from build123d import *

# Parameters (mm, degrees)
CYLINDER1852_R              = 3
CYLINDER1852_DEPTH          = 3
CYLINDER1853_R              = 3
CYLINDER1853_DEPTH          = 3
CYLINDER1854_R              = 3
CYLINDER1854_DEPTH          = 3
CYLINDER1851_R              = 3
CYLINDER1851_DEPTH          = 3
COMPOUND933_ROLL_ANGLE      = 90
COMPOUND933_PLACEMENT_ANGLE = 45
CYLINDER1848_R              = 1.5
CYLINDER1848_DEPTH          = 40
CYLINDER1850_R              = 1.5
CYLINDER1850_DEPTH          = 40
CYLINDER1849_R              = 1.5
CYLINDER1849_DEPTH          = 40
CYLINDER1847_R              = 1.5
CYLINDER1847_DEPTH          = 40
COMPOUND925_ROLL_ANGLE      = 90
COMPOUND925_PLACEMENT_ANGLE = 45
CYLINDER1867_R              = 12
CYLINDER1867_DEPTH          = 20
CYLINDER1866_R              = 2.5
CYLINDER1866_DEPTH          = 20
CYLINDER1864_R              = 2.5
CYLINDER1864_DEPTH          = 20
CYLINDER1863_R              = 2.5
CYLINDER1863_DEPTH          = 20
CYLINDER1865_R              = 2.5
CYLINDER1865_DEPTH          = 20
BOX324_W                    = 20
BOX324_H                    = 8
BOX324_DEPTH                = 3
BOX328_W                    = 20
BOX328_H                    = 8
BOX328_DEPTH                = 3
BOX330_W                    = 20
BOX330_H                    = 8
BOX330_DEPTH                = 3
BOX323_W                    = 20
BOX323_H                    = 8
BOX323_DEPTH                = 3
BOX329_W                    = 68
BOX329_H                    = 65
BOX329_DEPTH                = 8
CHAMFER014_SIZE             = 4


with BuildPart() as obj1:
    # Cylinder1852 → Cylinder1852 (new body)
    with BuildSketch(Plane(origin=(16, 140, 49), x_dir=(1, 0, 0), z_dir=(0, -1, 0))):
        Circle(CYLINDER1852_R)
    extrude(amount=CYLINDER1852_DEPTH)


with BuildPart() as obj2:
    # Cylinder1853 → Cylinder1853 (new body)
    with BuildSketch(Plane(origin=(-16, 140, 49), x_dir=(1, 0, 0), z_dir=(0, -1, 0))):
        Circle(CYLINDER1853_R)
    extrude(amount=CYLINDER1853_DEPTH)


with BuildPart() as obj3:
    # Cylinder1854 → Cylinder1854 (new body)
    with BuildSketch(Plane(origin=(0, 140, 33), x_dir=(1, 0, 0), z_dir=(0, -1, 0))):
        Circle(CYLINDER1854_R)
    extrude(amount=CYLINDER1854_DEPTH)


with BuildPart() as compound933:
    # Cylinder1851 → Cylinder1851 (new body)
    with BuildSketch(Plane(origin=(0, 140, 65), x_dir=(1, 0, 0), z_dir=(0, -1, 0))):
        Circle(CYLINDER1851_R)
    extrude(amount=CYLINDER1851_DEPTH)

    # Compound933: union obj1, obj2, obj3
    add(obj1.part)
    add(obj2.part)
    add(obj3.part)


with BuildPart() as compound933_1:
    # Compound933 roll: moved
    add(compound933.part.rotate(Axis((0, 0, 0), (1, 0, 0)), COMPOUND933_ROLL_ANGLE))


with BuildPart() as compound933_2:
    # Compound933 placement: moved
    add(compound933_1.part.moved(Location((-34.65, 34.65, -167))).rotate(Axis((-34.65, 34.65, -167), (0, 0, 1)), COMPOUND933_PLACEMENT_ANGLE))


with BuildPart() as obj4:
    # Cylinder1848 → Cylinder1848 (new body)
    with BuildSketch(Plane(origin=(16, 140, 49), x_dir=(1, 0, 0), z_dir=(0, -1, 0))):
        Circle(CYLINDER1848_R)
    extrude(amount=CYLINDER1848_DEPTH)


with BuildPart() as obj5:
    # Cylinder1850 → Cylinder1850 (new body)
    with BuildSketch(Plane(origin=(-16, 140, 49), x_dir=(1, 0, 0), z_dir=(0, -1, 0))):
        Circle(CYLINDER1850_R)
    extrude(amount=CYLINDER1850_DEPTH)


with BuildPart() as obj6:
    # Cylinder1849 → Cylinder1849 (new body)
    with BuildSketch(Plane(origin=(0, 140, 33), x_dir=(1, 0, 0), z_dir=(0, -1, 0))):
        Circle(CYLINDER1849_R)
    extrude(amount=CYLINDER1849_DEPTH)


with BuildPart() as compound925:
    # Cylinder1847 → Cylinder1847 (new body)
    with BuildSketch(Plane(origin=(0, 140, 65), x_dir=(1, 0, 0), z_dir=(0, -1, 0))):
        Circle(CYLINDER1847_R)
    extrude(amount=CYLINDER1847_DEPTH)

    # Compound925: union obj4, obj5, obj6
    add(obj4.part)
    add(obj5.part)
    add(obj6.part)


with BuildPart() as compound925_1:
    # Compound925 roll: moved
    add(compound925.part.rotate(Axis((0, 0, 0), (1, 0, 0)), COMPOUND925_ROLL_ANGLE))


with BuildPart() as compound925_2:
    # Compound925 placement: moved
    add(compound925_1.part.moved(Location((-34.65, 34.65, -144))).rotate(Axis((-34.65, 34.65, -144), (0, 0, 1)), COMPOUND925_PLACEMENT_ANGLE))


with BuildPart() as obj7:
    # Cylinder1867 → Cylinder1867 (new body)
    with BuildSketch(Plane.XY.offset(-39)):
        Circle(CYLINDER1867_R)
    extrude(amount=CYLINDER1867_DEPTH)


with BuildPart() as obj8:
    # Cylinder1866 → Cylinder1866 (new body)
    with BuildSketch(Plane(origin=(-23.55, 23.55, -34), x_dir=(1, 0, 0), z_dir=(0, 0, 1))):
        Circle(CYLINDER1866_R)
    extrude(amount=CYLINDER1866_DEPTH)


with BuildPart() as obj9:
    # Cylinder1864 → Cylinder1864 (new body)
    with BuildSketch(Plane(origin=(-23.55, -23.55, -34), x_dir=(1, 0, 0), z_dir=(0, 0, 1))):
        Circle(CYLINDER1864_R)
    extrude(amount=CYLINDER1864_DEPTH)


with BuildPart() as obj10:
    # Cylinder1863 → Cylinder1863 (new body)
    with BuildSketch(Plane(origin=(23.55, -23.55, -34), x_dir=(1, 0, 0), z_dir=(0, 0, 1))):
        Circle(CYLINDER1863_R)
    extrude(amount=CYLINDER1863_DEPTH)


with BuildPart() as compound931:
    # Cylinder1865 → Cylinder1865 (new body)
    with BuildSketch(Plane(origin=(23.55, 23.55, -34), x_dir=(1, 0, 0), z_dir=(0, 0, 1))):
        Circle(CYLINDER1865_R)
    extrude(amount=CYLINDER1865_DEPTH)

    # Compound931: union obj8, obj9, obj10
    add(obj8.part)
    add(obj9.part)
    add(obj10.part)


with BuildPart() as krychle324:
    # Box324 → Box324 (new body)
    with BuildSketch(Plane(origin=(17.55, -27.55, -28), x_dir=(1, 0, 0), z_dir=(0, 0, 1))):
        with Locations((10, 4)):
            Rectangle(BOX324_W, BOX324_H)
    extrude(amount=BOX324_DEPTH)


with BuildPart() as krychle328:
    # Box328 → Box328 (new body)
    with BuildSketch(Plane(origin=(-37.45, 19.55, -28), x_dir=(1, 0, 0), z_dir=(0, 0, 1))):
        with Locations((10, 4)):
            Rectangle(BOX328_W, BOX328_H)
    extrude(amount=BOX328_DEPTH)


with BuildPart() as krychle330:
    # Box330 → Box330 (new body)
    with BuildSketch(Plane(origin=(-37.45, -27.55, -28), x_dir=(1, 0, 0), z_dir=(0, 0, 1))):
        with Locations((10, 4)):
            Rectangle(BOX330_W, BOX330_H)
    extrude(amount=BOX330_DEPTH)


with BuildPart() as compound932:
    # Box323 → Box323 (new body)
    with BuildSketch(Plane(origin=(17.55, 19.55, -28), x_dir=(1, 0, 0), z_dir=(0, 0, 1))):
        with Locations((10, 4)):
            Rectangle(BOX323_W, BOX323_H)
    extrude(amount=BOX323_DEPTH)

    # Compound932: union Krychle324, Krychle328, Krychle330
    add(krychle324.part)
    add(krychle328.part)
    add(krychle330.part)


with BuildPart() as chamfer014:
    # Box329 → Box329 (new body)
    with BuildSketch(Plane(origin=(-34, -32, -30), x_dir=(1, 0, 0), z_dir=(0, 0, 1))):
        with Locations((34, 32.5)):
            Rectangle(BOX329_W, BOX329_H)
    extrude(amount=BOX329_DEPTH)

    # Cut314: cut Compound932
    add(compound932.part, mode=Mode.SUBTRACT)

    # Cut317: cut Compound931
    add(compound931.part, mode=Mode.SUBTRACT)

    # Cut315: cut obj7
    add(obj7.part, mode=Mode.SUBTRACT)

    # Cut319: cut Compound925
    add(compound925_2.part, mode=Mode.SUBTRACT)

    # Cut312: cut Compound933
    add(compound933_2.part, mode=Mode.SUBTRACT)

    # Chamfer014
    chamfer014_edges = [chamfer014.edges().sort_by_distance(p)[0] for p in [
        (0, -32, -22),
    ]]
    chamfer(chamfer014_edges, length=CHAMFER014_SIZE)


solid = chamfer014.part
Source: CAD feature listing. Evaluate the final solid. Frame: model axes, mm. A direction names the side the tool comes from. Round coordinates to 2 decimals unless told otherwise and drop trailing zeros. Loops run counter-clockwise (first coordinate to the right, second up) from the corner with the lowest first, then second, coordinate; pieces in that order, holes last. Notation, with made-up numbers: (40.5, 63) - (99.5, 63) arc R14 cw to (99.5, 83) - close; hole circle Ø5 at (9.5, -16). An arc over 180 degrees is marked (long way). Write item = value, one per line. Start each with the question number.
Item 1: Section query A-A on x = 0. Output: boundary loops of the cut face in (y, z).
Item 2: Mould query, pull axis Y, two halves, no side actions, for faces 5 (the face through (17.55, 23, -27)), 6 (the face through (-10.742, -9.926, -24.465)), 7 (the face through (0, -32, -28)), 8 (the face through (0, 33, -26)). Classes: released by +Y, released by -Y, zero draft, split by the parting line, or undercut.
Item 3: Section query B-B on y = -23.55. Output: boundary loops of the cut face in (x, z).
Item 4: Section query D-D on y = 1. Output: boundary loops of the cut face in (x, z), plus the area to 3 significant figures.
Item 5: First-contact query: pin 1 Ø3 at (x, y) = (23.55, 23.55) entering from +Z; pin 2 Ø8 at (x, y) = (11.31, 11.32) entering from +Z; pin 3 Ø0.9 at (y, z) = (-24, -27) entering from +X; pin 4 Ø1.5 at (y, z) = (24.5, -27) entering from -X. Flat tips, straight axial feed; report the tip coordinate or a pass-through.
Item 6: Material intervals for line 1 (Y direction, x = -23.55, z = -28.9); line 2 (X direction, y = -23.5, z = -22.75); line 3 (X direction, y = 0, z = -26), sorted ascending.
Item 7: Reachability of faces 1 (the face through (26, -19.55, -27)), 2 (the face through (13.14, -13.69, -28.48)), 3 (the face through (-28, -23, -28)), 4 (the face through (-24.09, 21.11, -23.52)) from +Z, -Z, +X, -X, +Y, -Y: full face, straight path, thin tool, end or side. Return the list, or none.
Item 8: Section query C-C on x = 28.5. Output: boundary loops of the cut face in (y, z).
Results list:
q1.outline = (-32, -30) - (-12, -30) - (-12, -22) - (-28, -22) - (-32, -26) - close; (12, -30) - (33, -30) - (33, -22) - (12, -22) - close
q2.face_5 = undercut
q2.face_6 = undercut
q2.face_7 = released by -Y
q2.face_8 = released by +Y
q3.outline = (-34, -30) - (-26.05, -30) - (-26.05, -28) - (-34, -28) - close; (-34, -25) - (-26.05, -25) - (-26.05, -22) - (-34, -22) - close; (-21.05, -30) - (21.05, -30) - (21.05, -28) - (17.55, -28) - (17.55, -25) - (21.05, -25) - (21.05, -22) - (-21.05, -22) - (-21.05, -25) - (-17.45, -25) - (-17.45, -28) - (-21.05, -28) - close; (26.05, -30) - (34, -30) - (34, -28) - (26.05, -28) - close; (26.05, -25) - (34, -25) - (34, -22) - (26.05, -22) - close
q4.outline = (-34, -30) - (-11.96, -30) - (-11.96, -22) - (-34, -22) - close; (11.96, -30) - (34, -30) - (34, -22) - (11.96, -22) - close
q4.area = 353 mm²
q5.pin_1 = through
q5.pin_2 = -22
q5.pin_3 = 17.55
q5.pin_4 = -17.45
q6.line_1 = -32 to -26.05, -21.05 to 21.05, 26.05 to 33
q6.line_2 = -34 to -26.05, -21.05 to 21.05, 26.05 to 34
q6.line_3 = -34 to -12, 12 to 34
q7.face_1 = +X
q7.face_2 = -Z
q7.face_3 = -X
q7.face_4 = +Z, -Z
q8.outline = (-32, -30) - (33, -30) - (33, -22) - (-28, -22) - (-32, -26) - close; hole (-27.55, -28) - (-19.55, -28) - (-19.55, -25) - (-27.55, -25) - close; hole (19.55, -28) - (27.55, -28) - (27.55, -25) - (19.55, -25) - close
